Can you work these out from the model? Positions are in its coordinate system, mm. A direction names the side the tool comes from. Coordinates: 2 decimals unless noted, no trailing zeros. Write each loop counter-clockwise with the first axis right and the second up, starting at its lowest first coordinate (ties: lowest second). Pieces come first, ordered by that corner, then holes.
```python
from build123d import *

# Parameters (mm, degrees)
F0_W     = 50
F0_H     = 300
F1_DEPTH = 50
F2_T     = -3
F3_R     = 5
F4_R     = 1
F5_R     = 5
F6_DEPTH = 50.001


with BuildPart() as f1:
    # F0 (on Front) → F1 (new body)
    with BuildSketch(Plane.XZ):
        with Locations((25, 150)):
            Rectangle(F0_W, F0_H)
    extrude(amount=F1_DEPTH)

    # F2
    f2_openings = [f1.faces().sort_by_distance(p)[0] for p in [
        (25, -25, 0),
        (25, 0, 150),
        (25, -25, 300),
    ]]
    offset(amount=F2_T, openings=f2_openings)

    # F3
    f3_edges = [f1.edges().sort_by_distance(p)[0] for p in [
        (50, -50, 150),
        (0, -50, 150),
    ]]
    fillet(f3_edges, radius=F3_R)

    # F4
    f4_edges = [f1.edges().sort_by_distance(p)[0] for p in [
        (47, 0, 150),
        (50, 0, 150),
        (3, 0, 150),
        (0, 0, 150),
        (3, -47, 150),
        (47, -47, 150),
    ]]
    fillet(f4_edges, radius=F4_R)

    # F5 (on face) → F6 (cut, through all)
    with BuildSketch(Plane(origin=(0, 0, 0), x_dir=(0, -1, 0), z_dir=(-1, 0, 0))):
        with Locations((20, 255)):
            Circle(F5_R)
        with Locations((20, 45)):
            Circle(F5_R)
    extrude(amount=-F6_DEPTH, mode=Mode.SUBTRACT)


solid = f1.part
```
1. If we section it at B-B, the plane y = -20: List the corners of the cut face in (x, z) for me, plus the area to 3 significant figures.
2. If we section it at C-C, the plane z = 255: List the corners of the cut face in (x, y) for me.
3. If we section it at D-D, the plane x = 17: List the corners of the cut face in (y, z) for me.
4. If I drill on L1, parallel to Z at x = 48, y = -20; L2, parallel to X at y = -2.5, z = 222; L3, parallel to Y at x = 36, z = 190.5, over which ranges is the centre line in solid material (lowest first)?
5. I'm going to push flat-ended pins straight in: P1, Ø1, axis at x = 33, z = 130, coming from the +Y side; P2, Ø8, axis at y = -20, z = 255, coming from the +X side. Where does each tip first touch, or does it pass through?
6. Which directions (+Z, -Z, +X, -X, +Y, -Y) give clear straight access to the entire face, cutting with the end or side of a thin tool? Please do faces 4 (the face through (50, -23, 148)), 5 (the face through (25, -47, 152)).
7. If we section it at A-A, the plane y = -33.5: List the corners of the cut face in (x, z) for me.
8. We'd pull the mould along X, two halves only. Please class faces 1 (the face through (25, -50, 152)), 2 (the face through (47, -23, 148)), 3 (the face through (1, -48, 152)): released by +X, released by -X, zero draft, split by the parting line, or undercut.
Answers:
1. outline: (0, 0) - (3, 0) - (3, 40) - (0, 40) - close; (0, 50) - (3, 50) - (3, 250) - (0, 250) - close; (0, 260) - (3, 260) - (3, 300) - (0, 300) - close; (47, 0) - (50, 0) - (50, 40) - (47, 40) - close; (47, 50) - (50, 50) - (50, 250) - (47, 250) - close; (47, 260) - (50, 260) - (50, 300) - (47, 300) - close
1. area: 1,680 mm2
2. outline: (0, -45) arc R5 ccw to (5, -50) - (45, -50) arc R5 ccw to (50, -45) - (50, -25) - (47, -25) - (47, -46) arc R1 cw to (46, -47) - (4, -47) arc R1 cw to (3, -46) - (3, -25) - (0, -25) - close; (0, -15) - (3, -15) - (3, -1) arc R1 ccw to (2, 0) - (1, 0) arc R1 ccw to (0, -1) - close; (47, -15) - (50, -15) - (50, -1) arc R1 ccw to (49, 0) - (48, 0) arc R1 ccw to (47, -1) - close
3. outline: (-50, 0) - (-47, 0) - (-47, 300) - (-50, 300) - close
4. L1: z = 0 to 40, 50 to 250, 260 to 300
4. L2: x = 0 to 3, 47 to 50
4. L3: y = -50 to -47
5. P1: stops at y = -47
5. P2: passes through
6. face 4: +Z, -Z, +X, +Y, -Y
6. face 5: +Z, -Z, +Y
7. outline: (0, 0) - (3, 0) - (3, 300) - (0, 300) - close; (47, 0) - (50, 0) - (50, 300) - (47, 300) - close
8. face 1: zero draft
8. face 2: undercut
8. face 3: released by -X
